```python
from build123d import *

# Parameters (mm, degrees)
SKETCH_3_R      = 1.5
EXTRUDE_1_DEPTH = 2


with BuildPart() as part:
    # 草图3 → 凸台-拉伸1 (new body)
    with BuildSketch(Plane.XY):
        Polygon((41, 20.009783315), (-41, 20.009783315), (-44, 20.009783315), (-44, 15.009783315), (-44, 5.009783315), (-44, 0.009783315), (-41, 0.009783315), (-41, -3.990216685), (-26.5, -3.990216685), (-26.5, 3.009783315), (26.5, 3.009783315), (26.5, -3.990216685), (41, -3.990216685), (41, 0.009783315), (44, 0.009783315), (44, 5.009783315), (44, 15.009783315), (44, 20.009783315), align=None)
        with Locations((-33.75, 15.509783315)):
            Circle(SKETCH_3_R, mode=Mode.SUBTRACT)
        with Locations((-33.75, 4.849783315)):
            Circle(SKETCH_3_R, mode=Mode.SUBTRACT)
        with Locations(Location((33.75, 4.849783315, 0), (0, 0, 180))):
            Circle(SKETCH_3_R, mode=Mode.SUBTRACT)
        with Locations(Location((33.75, 15.509783315, 0), (0, 0, 180))):
            Circle(SKETCH_3_R, mode=Mode.SUBTRACT)
        with BuildLine():
            Line((37.1, -2.090216685), (29.9, -2.090216685))
            ThreePointArc((29.9, -2.090216685), (29.444365081, -0.990216685), (29.9, 0.109783315))
            Line((29.9, 0.109783315), (37.1, 0.109783315))
            Line((37.1, 0.109783315), (37.1, -2.090216685))
        make_face(mode=Mode.SUBTRACT)
        with BuildLine():
            Line((-37.1, 0.109783315), (-29.9, 0.109783315))
            ThreePointArc((-29.9, 0.109783315), (-29.444365081, -0.990216685), (-29.9, -2.090216685))
            Line((-29.9, -2.090216685), (-37.1, -2.090216685))
            Line((-37.1, -2.090216685), (-37.1, 0.109783315))
        make_face(mode=Mode.SUBTRACT)
        with BuildLine():
            Line((-43.1, 15.049783315), (-43.1, 4.849783315))
            Line((-43.1, 4.849783315), (-40.9, 4.849783315))
            Line((-40.9, 4.849783315), (-40.9, 15.049783315))
            ThreePointArc((-40.9, 15.049783315), (-42, 15.505418233), (-43.1, 15.049783315))
        make_face(mode=Mode.SUBTRACT)
        with BuildLine():
            Line((40.9, 15.049783315), (40.9, 4.849783315))
            Line((40.9, 4.849783315), (43.1, 4.849783315))
            Line((43.1, 4.849783315), (43.1, 15.049783315))
            ThreePointArc((43.1, 15.049783315), (42, 15.505418233), (40.9, 15.049783315))
        make_face(mode=Mode.SUBTRACT)
    extrude(amount=EXTRUDE_1_DEPTH)


solid = part.part
```
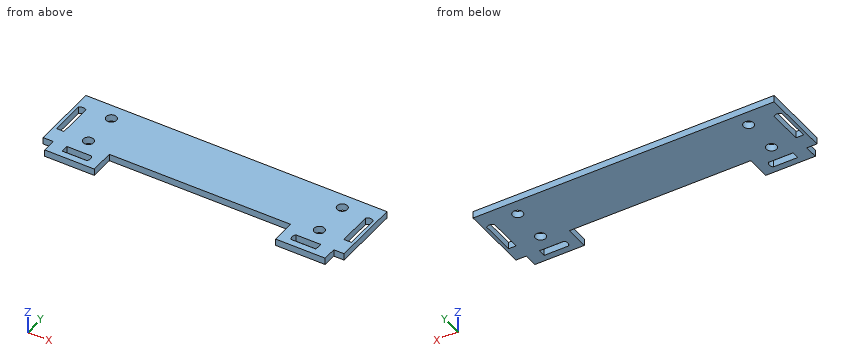
Geometry check sheet. Reference: the model listing, model coordinates, mm. Coordinates: 2 decimals unless noted, no trailing zeros. Order: outer loops, then holes, each group sorted by start corner. A loop starts at its lowest first (then second) coordinate and runs counter-clockwise, first axis right, second up. Notation, with made-up numbers: (51, 75) - (106, 75) arc R20 ccw to (106, 98) - close; hole circle Ø1 at (59.25, 58.5). An arc over 180 degrees is marked (long way). Answer in a Markdown table with one row per item. Add a question column.
1. Gauge pin test, flat ends, axial feed: pin 1 Ø0.6 at (x, z) = (-43, 1.5) entering from -Y; pin 2 Ø2.5 at (x, y) = (-33.75, 4.85) entering from +Z; pin 3 Ø0.6 at (y, z) = (-3, 1.5) entering from +X; pin 4 Ø3.5 at (x, y) = (33.75, 4.85) entering from -Z. Record the tip position at first contact, or that the pin passes through.
2. Material ranges on L1, parallel to X at y = 8.75, z = 0.2; L2, parallel to Y at x = 33.75, z = 1.2; L3, parallel to X at y = -1, z = 1.95, recorded low to high. Write a range as [from, to].
3. Section check B-B (x = -33.75). Enter the section's corners in (y, z).
4. Section check D-D (x = 14). Enter the section's corners in (y, z).
5. Section check C-C (z = 1). Give the number of separate pieces and of enclosed holes in the cut face, plus the area to 3 significant figures.
6. Section check A-A (y = 11.5). Enter the section's corners in (x, z).
Data:
| question | item | result |
|---|---|---|
| 1 | pin 1 | stops at y = 0.01 |
| 1 | pin 2 | passes through |
| 1 | pin 3 | stops at x = 41 |
| 1 | pin 4 | stops at z = 0 |
| 2 | L1 | x = [-44, -43.1], [-40.9, 40.9], [43.1, 44] |
| 2 | L2 | y = [-3.99, -2.09], [0.11, 3.35], [6.35, 14.01], [17.01, 20.01] |
| 2 | L3 | x = [-41, -37.1], [-29.44, -26.5], [26.5, 29.44], [37.1, 41] |
| 3 | outline | (-3.99, 0) - (-2.09, 0) - (-2.09, 2) - (-3.99, 2) - close; (0.11, 0) - (3.35, 0) - (3.35, 2) - (0.11, 2) - close; (6.35, 0) - (14.01, 0) - (14.01, 2) - (6.35, 2) - close; (17.01, 0) - (20.01, 0) - (20.01, 2) - (17.01, 2) - close |
| 4 | outline | (3.01, 0) - (20.01, 0) - (20.01, 2) - (3.01, 2) - close |
| 5 | separate pieces | 1 |
| 5 | enclosed holes | 8 |
| 5 | area | 1,610 mm² |
| 6 | outline | (-44, 0) - (-43.1, 0) - (-43.1, 2) - (-44, 2) - close; (-40.9, 0) - (40.9, 0) - (40.9, 2) - (-40.9, 2) - close; (43.1, 0) - (44, 0) - (44, 2) - (43.1, 2) - close |
